Verification items for the finished model (mm, model axes). Round coordinates to 2 decimals unless told otherwise and drop trailing zeros. Order: outer loops, then holes, each group sorted by start corner. A loop starts at its lowest first (then second) coordinate and runs counter-clockwise, first axis right, second up. Notation, with made-up numbers: (78, 42.5) -> (104, 42.5) arc R21 ccw to (104, 76.5) -> close; hole circle Ø6 at (59.5, -18.75). An arc over 180 degrees is marked (long way). Put each result on its own line as item: value.
```python
from build123d import *

# Parameters (mm, degrees)
F0_R     = 25.4
F0_R_2   = 23.8125
F1_DEPTH = 304.8
F2_R     = 3.175
F3_DEPTH = 25.4
F4_R     = 3.175
F5_DEPTH = 25.4


with BuildPart() as f1:
    # F0 (on Front) → F1 (new body, symmetric)
    with BuildSketch(Plane.XZ):
        Circle(F0_R)
        Circle(F0_R_2, mode=Mode.SUBTRACT)
    extrude(amount=F1_DEPTH, both=True)

    # F2 (on Right) → F3 (cut, symmetric)
    with BuildSketch(Plane.YZ):
        with Locations((-279.4, 0)):
            Circle(F2_R)
        with Locations((292.1, 0)):
            Circle(F2_R)
    extrude(amount=F3_DEPTH, both=True, mode=Mode.SUBTRACT)

    # F4 (on Top) → F5 (cut, symmetric)
    with BuildSketch(Plane.XY):
        with Locations((0, 266.7)):
            Circle(F4_R)
    extrude(amount=F5_DEPTH, both=True, mode=Mode.SUBTRACT)


solid = f1.part
```
Item 1: Release check for a two-part mould opening along X. For faces 1 (the face through (-23, -304.8, -7)), 2 (the face through (-18.897, 4.267, -14.49)), 3 (the face through (-5.506, -4.267, -24.796)) record: pulls with the +X half, pulls with the -X half, needs draft (parallel to the pull), parting line crosses it, or undercut.
Geometry check:
face 1: needs draft
face 2: undercut
face 3: parting line crosses it
Item 2: Sectioned sample at B-B, the plane x = 18.5. Record the boundary of the cut face in (y, z), then the cut area to 3 significant figures.
Geometry check:
outline: (-304.8, -17.4) -> (304.8, -17.4) -> (304.8, -14.99) -> (-304.8, -14.99) -> close; (-304.8, 14.99) -> (304.8, 14.99) -> (304.8, 17.4) -> (-304.8, 17.4) -> close
area: 2,940 mm2
Item 3: Material ranges on line 1 along Y through (x, z) = (24, 0) (3 decimals); line 2 along X through (y, z) = (-106.5, 0.5), recorded low to high.
Geometry check:
line 1: -304.8 to -282.575, -276.225 to 288.925, 295.275 to 304.8
line 2: -25.4 to -23.81, 23.81 to 25.4
Item 4: Depth check by flat-ended pin: pin 1 Ø3 at (y, z) = (-118, 4) entering from -X; pin 2 Ø8 at (x, y) = (-0.5, -183.5) entering from +Z; pin 3 Ø5 at (x, y) = (0, 266.7) entering from +Z. Enter the tip coordinate at first touch or a pass-through.
Geometry check:
pin 1: x = -25.28
pin 2: z = 25.4
pin 3: through
Item 5: Sectioned sample at A-A, the plane z = 10.5. Record the boundary of the cut face in (x, y), then the cut area to 3 significant figures.
Geometry check:
outline: (-23.13, -304.8) -> (-21.37, -304.8) -> (-21.37, 304.8) -> (-23.13, 304.8) -> close; (21.37, -304.8) -> (23.13, -304.8) -> (23.13, 304.8) -> (21.37, 304.8) -> close
area: 2,140 mm2
Item 6: Sectioned sample at C-C, the plane y = -32. Record the boundary of the cut face in (x, z) (1 decimal).
Geometry check:
outline: circle Ø50.8 at (0, 0); hole circle Ø47.6 at (0, 0)
